Geometry check sheet. Reference: the model listing, model coordinates, mm. Face numbers are marked on the shaded views. A direction names the side the tool comes from. Coordinates: 2 decimals unless noted, no trailing zeros. Order: outer loops, then holes, each group sorted by start corner. A loop starts at its lowest first (then second) coordinate and runs counter-clockwise, first axis right, second up. Notation, with made-up numbers: (-25.5, 22) - (11.5, 22) arc R25 cw to (11.5, 34) - close; hole circle Ø6 at (32, 24). An arc over 180 degrees is marked (long way). Put each result on its own line as item: value.
from build123d import *

# Parameters (mm, degrees)
F1_DEPTH = 2.5
F2_R     = 0.7249372234
F3_DEPTH = 2.5
F5_DEPTH = 0.7


with BuildPart() as f1:
    # F0 (on Front) → F1 (new body)
    with BuildSketch(Plane.XZ):
        Polygon((-9.4160782173, 4.8845554702), (-12.13010028, -2.4174565915), (-7.8005888499, -2.4174565915), (-6.7666755058, 0), (-4.8927078024, -2.4174565915), (3.4432173707, -2.6133938689), (6.6945207968, 0), (6.7388154566, -2.6133938689), (10.5981117284, -2.6133938689), (13.2007738575, 0.5550436326), (13.0135210928, -2.6133938689), (16.9487092644, -2.5466959924), (17.65952399, 4.9491748214), (13.846969232, 4.8845554702), (11.5687668393, 2.1111098447), (11.5206642076, 4.9491748214), (7.7081094496, 4.8845554702), (3.7663155235, 1.0073808953), (5.3818048909, 5.9184683487), (11.2621868029, 5.9184683487), (11.8437623605, 7.1462406777), (-4.1818926111, 7.1462406777), (-4.6988492832, 5.9830881655), (0.8584343595, 5.9830881655), (-1.5324898995, -0.8019671077), (-3.277218435, 1.9766744226), (0, 4.8845554702), (-3.0833596829, 4.8845554702), (-6.3789580017, 2.1059135906), (-5.2158059552, 4.8845554702), align=None)
    extrude(amount=F1_DEPTH)

    # F2 (on face) → F3 (cut, through all)
    with BuildSketch(Plane.XZ.offset(2.5)):
        with Locations((-10.5334725231, -1.3533922611)):
            Circle(F2_R)
    extrude(amount=-F3_DEPTH, mode=Mode.SUBTRACT)

    # F4 (on face) → F5 (join)
    with BuildSketch(Plane.XZ.offset(2.5)):
        Polygon((11.129762046, 6.9781923667), (-3.4941763151, 6.9781923667), (-3.7754920777, 6.9781923667), (-3.8937546778, 6.9781923667), (-4.1818926111, 6.1621805653), (-4.0636300109, 6.1621805653), (-1.2187248794, 6.1621805653), (1.055368688, 6.1621805653), (1.1777002364, 6.1621805653), (-0.993734838, 0), (-1.5324898995, -1.3987065759), (-1.8525599505, -2.2296669082), (2.4666503559, -2.2296669082), (3.4364298917, 0.7184627466), (5.2153817378, 6.1621805653), (5.4596047848, 6.1621805653), (10.9740488697, 6.1621805653), (11.2621868029, 6.9781923667), align=None)
    extrude(amount=F5_DEPTH)


solid = f1.part
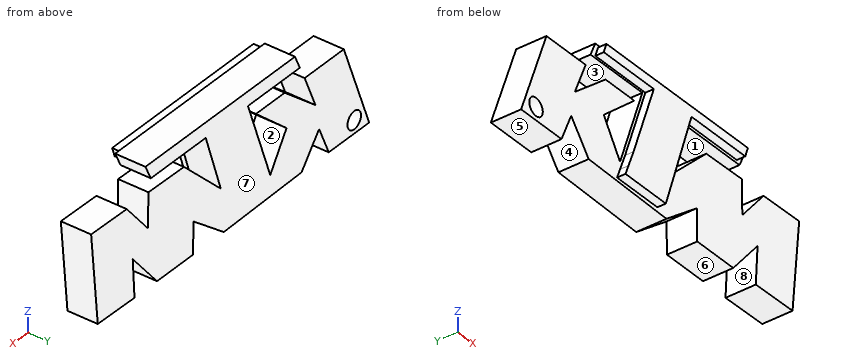
Q1. Section check C-C on x = -2.25. Record the boundary of the cut face in (y, z), then the cut area to 3 significant figures.
Answer block:
outline: (-3.2, 6.16) - (-2.5, 6.16) - (-2.5, 5.98) - (0, 5.98) - (0, 7.15) - (-2.5, 7.15) - (-2.5, 6.98) - (-3.2, 6.98) - close; (-2.5, -2.48) - (0, -2.48) - (0, 0.34) - (-2.5, 0.34) - close; (-2.5, 2.89) - (0, 2.89) - (0, 4.88) - (-2.5, 4.88) - close
area: 15.5 mm^2
Q2. Draft check along Z on the marked faces 6, 7 and 8. Enter one of: pulls with the +Z half, pulls with the -Z half, needs draft (parallel to the pull), parting line crosses it, or undercut.
Answer block:
face 6: pulls with the -Z half
face 7: needs draft
face 8: undercut
Q3. Depth check by flat-ended pin: pin 1 Ø0.8 at (x, y) = (-9.5, -1.5) entering from -Z; pin 2 Ø3 at (x, z) = (8, -1.5) entering from +Y; pin 3 Ø0.8 at (x, y) = (-7, -1.5) entering from +Z; pin 4 Ø5 at (x, z) = (7, 2.5) entering from -Y. Enter the tip coordinate at first touch or a pass-through.
Answer block:
pin 1: stops at z = -2.42
pin 2: stops at y = 0
pin 3: stops at z = 4.88
pin 4: stops at y = -2.5
Q4. Section check D-D on z = 3.25. Record the boundary of the cut face in (x, y), then the cut area to 3 significant figures.
Answer block:
outline: (-10.02, -2.5) - (-5.9, -2.5) - (-5.9, 0) - (-10.02, 0) - close; (-5.02, -2.5) - (-1.84, -2.5) - (-1.84, 0) - (-5.02, 0) - close; (-0.1, -2.5) - (0.15, -2.5) - (0.15, -3.2) - (4.26, -3.2) - (4.26, -2.5) - (4.5, -2.5) - (4.5, 0) - (-0.1, 0) - close; (6.05, -2.5) - (11.55, -2.5) - (11.55, 0) - (6.05, 0) - close; (12.5, -2.5) - (17.5, -2.5) - (17.5, 0) - (12.5, 0) - close
area: 58.9 mm^2
Q5. Section check B-B on x = 4.25. Record the boundary of the cut face in (y, z).
Answer block:
outline: (-3.2, 3.21) - (-2.5, 3.21) - (-2.5, 2.48) - (0, 2.48) - (0, 7.15) - (-2.5, 7.15) - (-2.5, 6.98) - (-3.2, 6.98) - close; (-2.5, -1.96) - (0, -1.96) - (0, 1.48) - (-2.5, 1.48) - close
Q6. Access from +Z, -Z, +X, -X, +Y, -Y to the whole of each face (thin tool, end or side, straight path). Record for the marked faces 1, 2, 3, 4 and 5.
Answer block:
face 1: +X, +Y, -Y
face 2: +Y, -Y
face 3: -X, +Y, -Y
face 4: -Z, +Y, -Y
face 5: -Z, -X, +Y, -Y
Q7. Thickness scan on L1, parallel to X at y = -1.15, z = 3; L2, parallel to X at y = -1.9, z = 4; L3, parallel to X at y = -0.35, z = 0.25. Record the ranges inside material, lowest first. Write a range as [from, to].
Answer block:
L1: x = [-10.12, -6], [-5.32, -2.12], [-0.19, 4.42], [5.79, 11.55], [12.3, 17.47]
L2: x = [-9.74, -5.59], [-4.13, -1], [0.16, 4.75], [6.81, 11.54], [13.12, 17.57]
L3: x = [-11.14, -2.19], [-1.16, 12.95], [13.18, 17.21]
Q8. Section check A-A on y = -2.9. Record the boundary of the cut face in (x, z).
Answer block:
outline: (-4.18, 6.16) - (1.18, 6.16) - (-0.99, 0) - (-1.85, -2.23) - (2.47, -2.23) - (3.44, 0.72) - (5.22, 6.16) - (10.97, 6.16) - (11.26, 6.98) - (-3.89, 6.98) - close
